from build123d import *

# Parameters (mm, degrees)
SKETCH_2_R = 1.5


with BuildPart() as part:
    # По траектории1: sweep along a path in Эскиз1
    with BuildLine(Plane(origin=(0, 0, 0), x_dir=(0, 0, -1), z_dir=(1, 0, 0))) as sweep_1_path:
        Line((0, 0), (0, 45))
        ThreePointArc((0, 45), (-2.928932188, 52.071067812), (-10, 55))
        Line((-10, 55), (-20, 55))
        ThreePointArc((-20, 55), (-27.071067812, 52.071067812), (-30, 45))
        Line((-30, 45), (-30, 25))
    # Эскиз2 → По траектории1 (sweep)
    with BuildSketch(Plane(origin=(0, 0, 0), x_dir=(1, 0, 0), z_dir=(0, 1, 0))):
        Circle(SKETCH_2_R)
    sweep(path=sweep_1_path.line)

    # Зеркальное отражение1: part across plane


with BuildPart() as part_1:
    add(part.part)
    add(part.part.mirror(Plane.ZX))


solid = part_1.part
Read the model definition and answer for the solid it produces. Units are mm, in the model's axes. A direction names the side the tool comes from. Coordinates: 2 decimals unless noted, no trailing zeros. Write each loop counter-clockwise with the first axis right and the second up, starting at its lowest first coordinate (ties: lowest second). Pieces come first, ordered by that corner, then holes. Notation, with made-up numbers: (-31, 22.25) -> (-24, 22.25) arc R20 ccw to (-24, 46.25) -> close; hole circle Ø2 at (58.5, -29.75). An arc over 180 degrees is marked (long way). Return JSON: item names as keys, results as strings.
(1) For a pull along Z with two mould halves and no side action, classify faces 1 (the cylindrical face through (-1.2, 54.1, 15.1)), 2 (the flat face through (0, 25, 30)) as pulls with the +Z half, pulls with the -Z half, needs draft (parallel to the pull), parting line crosses it, or undercut.
Answers below:
{"face 1": "undercut", "face 2": "needs draft"}
(2) The part is cut by section B-B on y = -27. Give the vertices of the cut face in (x, z), then the cut area to 3 significant figures.
Answers below:
{"outline": "circle Ø3 at (0, 0); circle Ø3 at (0, 30)", "area": "14.1 mm^2"}
(3) The part is cut by section C-C on y = 3. Give the vertices of the cut face in (x, z), then the cut area to 3 significant figures.
Answers below:
{"outline": "circle Ø3 at (0, 0)", "area": "7.07 mm^2"}
(4) The part is cut by section A-A on x = -0.9. Give the vertices of the cut face in (y, z), then the cut area to 3 significant figures.
Answers below:
{"outline": "(-56.2, 10) arc R11.2 ccw to (-45, -1.2) -> (45, -1.2) arc R11.2 ccw to (56.2, 10) -> (56.2, 20) arc R11.2 ccw to (45, 31.2) -> (25, 31.2) -> (25, 28.8) -> (45, 28.8) arc R8.8 cw to (53.8, 20) -> (53.8, 10) arc R8.8 cw to (45, 1.2) -> (-45, 1.2) arc R8.8 cw to (-53.8, 10) -> (-53.8, 20) arc R8.8 cw to (-45, 28.8) -> (-25, 28.8) -> (-25, 31.2) -> (-45, 31.2) arc R11.2 ccw to (-56.2, 20) -> close", "area": "511 mm^2"}
(5) Which of the six approach directions +Z, -Z, +X, -X, +Y, -Y give full straight-line access (tool end or side, diameter ignored) to faces 3 (the flat face through (0, -25, 30)), 4 (the cylindrical face through (-1.2, -54.1, 15.1))?
Answers below:
{"face 3": "+Z, +X, -X", "face 4": "none"}
(6) Consider line 1 along Z through (x, y) = (-0.15, -33); line 2 along Y through (x, z) = (0.15, 15); line 3 along Y through (x, z) = (1.25, 23). Determine where each line is inside the solid, lowest interval first. Write a range as from..to.
Answers below:
{"line 1": "-1.49..1.49, 28.51..31.49", "line 2": "-56.49..-53.51, 53.51..56.49", "line 3": "-55.41..-53.67, 53.67..55.41"}
